```python
from build123d import *

# Parameters (mm, degrees)
F1_DEPTH = 86.11
F2_R     = 5
F3_R     = 5
F4_R     = 5


# Not quite as in the source:
# - the dataset's text gives a spline's control points without its knots; the knots are read off the source's solid


with BuildPart() as f1:
    # F0 (on Top) → F1 (new body)
    with BuildSketch(Plane.XY):
        with BuildLine():
            add(Edge.make_bspline(
                [(-29.23, -10.585), (-17.4530325989, -10.3312646709), (-14.3938385965, -9.9964864644), (-4.3826738853, -13.2963216573)],
                knots=[0, 0, 0, 0, 24.9948170664, 24.9948170664, 24.9948170664, 24.9948170664], degree=3))
            ThreePointArc((-4.3826738853, -13.2963216573), (14, 0), (-4.3826738853, 13.2963216573))
            add(Edge.make_bspline(
                [(-29.23, 10.585), (-17.4530325989, 10.3312646709), (-14.3938385965, 9.9964864644), (-4.3826738853, 13.2963216573)],
                knots=[0, 0, 0, 0, 24.9948170664, 24.9948170664, 24.9948170664, 24.9948170664], degree=3))
            Line((-29.23, 10.585), (-29.23, 7.5843010349))
            add(Edge.make_bspline(
                [(-29.2300000018, 7.5843009524), (-26.3264289999, 7.5214949579), (-22.7397747479, 7.4189906626), (-18.7158912708, 7.4405712538), (-15.8829489535, 7.5882179461), (-13.0899113875, 7.919906296), (-10.2045998481, 8.4774191522), (-7.0815280556, 9.2907869197), (-4.7236583696, 10.0251594583), (-3.443529459, 10.447109806)],
                knots=[0.0018385431, 0.0018385431, 0.0018385431, 0.0018385431, 0.25, 0.375, 0.5, 0.625, 0.75, 0.875, 1, 1, 1, 1], degree=3))
            ThreePointArc((-3.443529459, 10.447109806), (10.9999999288, 0), (-3.443529459, -10.447109806))
            add(Edge.make_bspline(
                [(-29.2300000018, -7.5843009524), (-26.3264289999, -7.5214949579), (-22.7397747479, -7.4189906626), (-18.7158912708, -7.4405712538), (-15.8829489535, -7.5882179461), (-13.0899113875, -7.919906296), (-10.2045998481, -8.4774191522), (-7.0815280556, -9.2907869197), (-4.7236583696, -10.0251594583), (-3.443529459, -10.447109806)],
                knots=[0.0018385431, 0.0018385431, 0.0018385431, 0.0018385431, 0.25, 0.375, 0.5, 0.625, 0.75, 0.875, 1, 1, 1, 1], degree=3))
            Line((-29.23, -7.5843010349), (-29.23, -10.585))
        make_face()
    extrude(amount=F1_DEPTH)

    # F2
    f2_edges = [f1.edges().sort_by_distance(p)[0] for p in [
        (-29.23, -9.084651, 0),
    ]]
    fillet(f2_edges, radius=F2_R)

    # F3
    f3_edges = [f1.edges().sort_by_distance(p)[0] for p in [
        (-29.23, 9.084651, 0),
    ]]
    fillet(f3_edges, radius=F3_R)

    # F4
    f4_edges = [f1.edges().sort_by_distance(p)[0] for p in [
        (-29.23, -9.084651, 86.11),
        (-29.23, 9.084651, 86.11),
    ]]
    fillet(f4_edges, radius=F4_R)


solid = f1.part
```
Model file for the job. Use its own axes, mm. Coordinates: 2 decimals unless noted, no trailing zeros. Order: outer loops, then holes, each group sorted by start corner. A loop starts at its lowest first (then second) coordinate and runs counter-clockwise, first axis right, second up. Notation, with made-up numbers: (20.5, -36) -> (73.5, -36) arc R14 cw to (73.5, -22) -> close; hole circle Ø2 at (26.25, 37). An arc over 180 degrees is marked (long way). Answer as a JSON object with one key per item and string values. Group by question number.
1) Cut at B-B, the plane y = 0. Write the cut outline in (x, z).
2) Cut at A-A, the plane x = 0. Write the cut outline in (y, z), then the cut area to 3 significant figures.
3) Cut at D-D, the plane y = 4. Write the cut outline in (x, z).
4) Cut at C-C, the plane x = 10. Write the cut outline in (y, z).
5) Drill centre lines: L1, parallel to Y at x = 0, z = 44; L2, parallel to Y at x = -8, z = 19; L3, parallel to X at y = -7, z = 22. Where is each one in solid material? Low to high.
6) Flat gauge pins, fed straight in: pin 1 (1.5 mm diameter, centred on x = -1, z = 49, fed in from +Y); pin 2 (3 mm diameter, centred on y = -5, z = 67, fed in from +X); pin 3 (5 mm diameter, centred on y = 7, z = 19, fed in from +X). Where does each tip first touch, or does it go through?
7) Pull direction Y, two halves, no side cores. Call faces 1 (the face through (11, 0, 42)), 2 (the face through (14, 0, 42)), 3 (the face through (-29.23, -9, 43)): +Y half, -Y half, draft (parallel to the pull), parting line (faces both ways), or undercut.
Check values:
{
 "1": {"outline": "(11, 0) -> (14, 0) -> (14, 86.11) -> (11, 86.11) -> close"},
 "2": {"outline": "(-14, 0) -> (-11, 0) -> (-11, 86.11) -> (-14, 86.11) -> close; (11, 0) -> (14, 0) -> (14, 86.11) -> (11, 86.11) -> close", "area": "517 mm²"},
 "3": {"outline": "(10.25, 0) -> (13.42, 0) -> (13.42, 86.11) -> (10.25, 86.11) -> close"},
 "4": {"outline": "(-9.8, 0) -> (-4.58, 0) -> (-4.58, 86.11) -> (-9.8, 86.11) -> close; (4.58, 0) -> (9.8, 0) -> (9.8, 86.11) -> (4.58, 86.11) -> close"},
 "5": {"L1": "y = -14 to -11, 11 to 14", "L2": "y = -12.18 to -9.06, 9.06 to 12.18", "L3": "x = 8.49 to 12.12"},
 "6": {"pin 1": "stops at y = 14", "pin 2": "stops at x = 13.56", "pin 3": "stops at x = 13.26"},
 "7": {"face 1": "undercut", "face 2": "parting line", "face 3": "draft"}
}
